Can you work these out from the drawing? Everything is in mm from the part's minimum corner. A direction names the side the tool comes from. Coordinates: 2 decimals unless noted, no trailing zeros. Write each loop counter-clockwise with the first axis right and the second up, starting at its lowest first coordinate (ties: lowest second). Pieces come first, ordered by that corner, then holes.
(1) Please list where these lines run through material, in increasing order: probe 1 along X at (y, z) = (14.35, 5); probe 2 along Z at (x, y) = (57, 2.6); probe 3 along Y at (x, z) = (54.5, 7).
(2) Thinking about a two-plate mould opening in X: for the marked faces 4, 5 and 6, which applies, released by +X, released by -X, zero draft, split by the parting line, or undercut?
(3) Which directions (+Z, -Z, +X, -X, +Y, -Y) give clear straight access to the entire face, cutting with the end or side of a thin tool? Please do the marked faces 1, 2 and 3.
(4) Imagine slicing it at C-C, the plane y = 14.25. List the corners of the cut face in (x, z) for me, plus the area to 3 significant figures.
(5) For pin 1 Ø5 at (x, z) = (10, 5) entering from +Y; pin 2 Ø1 at (y, z) = (5, 7.5) entering from -X; pin 3 Ø3.5 at (x, z) = (57, 5) entering from +Y; pin 4 Ø3 at (x, z) = (22, 3.5) entering from -Y, each with a flat end and sliding along its axis, tell me the tip position at first contact or that it passes through.
(6) Imagine slicing it at B-B, the plane x = 57. List the corners of the cut face in (y, z) for me, plus the area to 3 significant figures.
(7) Imagine slicing it at D-D, the plane z = 2. List the corners of the cut face in (x, y) for me, plus the area to 3 significant figures.
(8) Imagine slicing it at A-A, the plane z = 5. List the corners of the cut face in (x, y) for me, plus the area to 3 significant figures.
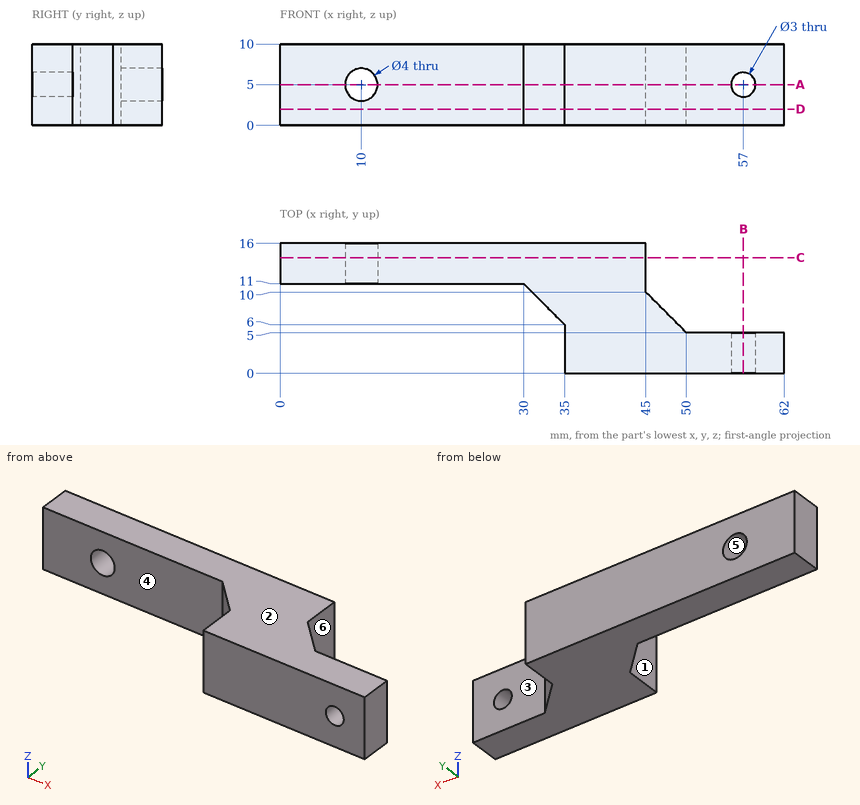
Recorded:
1. probe 1: x = 0 to 8, 12 to 45
1. probe 2: z = 0 to 3.5, 6.5 to 10
1. probe 3: y = 0 to 5
2. face 4: zero draft
2. face 5: undercut
2. face 6: released by +X
3. face 1: +Z, -Z, -X, -Y
3. face 2: +Z, +X, -X, +Y, -Y
3. face 3: +Z, -Z, +X, +Y
4. outline: (0, 0) - (45, 0) - (45, 10) - (0, 10) - close; hole circle Ø4 at (10, 5)
4. area: 437 mm2
5. pin 1: stops at y = 16
5. pin 2: stops at x = 35
5. pin 3: stops at y = 5
5. pin 4: stops at y = 11
6. outline: (0, 0) - (5, 0) - (5, 3.5) - (0, 3.5) - close; (0, 6.5) - (5, 6.5) - (5, 10) - (0, 10) - close
6. area: 35.0 mm2
7. outline: (0, 11) - (30, 11) - (35, 6) - (35, 0) - (62, 0) - (62, 5) - (50, 5) - (45, 10) - (45, 16) - (0, 16) - close
7. area: 445 mm2
8. outline: (0, 11) - (8, 11) - (8, 16) - (0, 16) - close; (12, 11) - (30, 11) - (35, 6) - (35, 0) - (55.5, 0) - (55.5, 5) - (50, 5) - (45, 10) - (45, 16) - (12, 16) - close; (58.5, 0) - (62, 0) - (62, 5) - (58.5, 5) - close
8. area: 410 mm2
